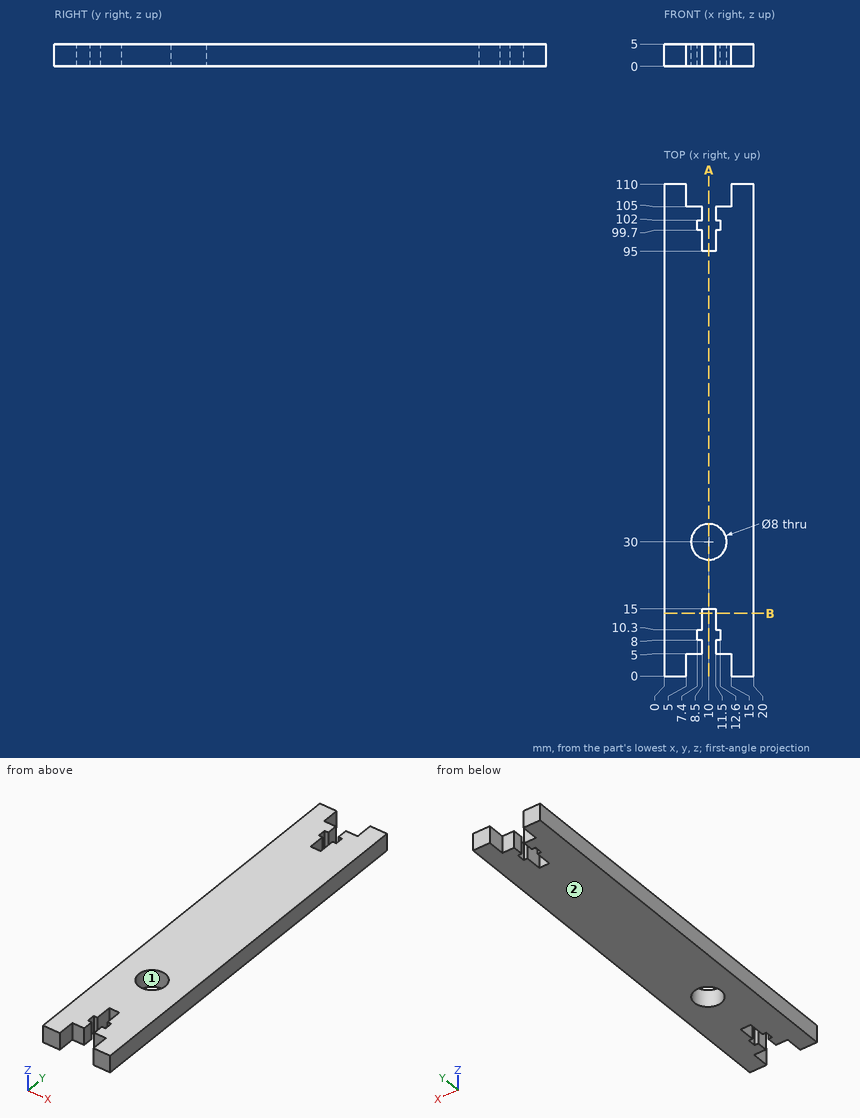
Geometry: see drawing. Coordinates: mm, zero at the bounding-box minimum. Coordinates: 2 decimals unless noted, no trailing zeros. Write each loop counter-clockwise with the first axis right and the second up, starting at its lowest first coordinate (ties: lowest second). Pieces come first, ordered by that corner, then holes.
1) Mould query, pull axis X, two halves, no side actions, for the marked faces 1 and 2. Classes: pulls with the +X half, pulls with the -X half, needs draft (parallel to the pull), parting line crosses it, or undercut.
2) Section A-A on x = 10. Output: boundary loops of the cut face in (y, z).
3) Pin query (flat end, axial travel): pin 1 Ø0.9 at (x, z) = (8, 3.5) entering from -Y; pin 2 Ø6.5 at (x, y) = (10, 30) entering from -Z; pin 3 Ø1 at (x, z) = (13, 2.5) entering from +Y. Return the tip coordinate at first contact, or that it passes through.
4) Section B-B on y = 14. Output: boundary loops of the cut face in (x, z).
5) Material intervals for line 1 along X through (y, z) = (10, 2.3); line 2 along Y through (x, z) = (10, 2.9); line 3 along X through (y, z) = (13.5, 2.4), sorted ascending.
Check result:
1. face 1: undercut
1. face 2: needs draft
2. outline: (15, 0) - (26, 0) - (26, 5) - (15, 5) - close; (34, 0) - (95, 0) - (95, 5) - (34, 5) - close
3. pin 1: stops at y = 5
3. pin 2: passes through
3. pin 3: stops at y = 105
4. outline: (0, 0) - (8.5, 0) - (8.5, 5) - (0, 5) - close; (11.5, 0) - (20, 0) - (20, 5) - (11.5, 5) - close
5. line 1: x = 0 to 7.4, 12.6 to 20
5. line 2: y = 15 to 26, 34 to 95
5. line 3: x = 0 to 8.5, 11.5 to 20
